Here's the drawing with two shaded views (mm, measured from the low corner). I have some questions. A direction names the side the tool comes from. Give positions to 0.01 mm unless a question says otherwise; leave off trailing zeros. Order: outer loops, then holes, each group sorted by start corner. A loop starts at its lowest first (then second) coordinate and runs counter-clockwise, first axis right, second up. Notation, with made-up numbers: M 52,25.25 L 80,25.25 A26 ccw 80,63.25 Z; hole C -32.75,-17 d11. An arc over 180 degrees is marked long. Write each question's results on one line, items separated by ' | '.
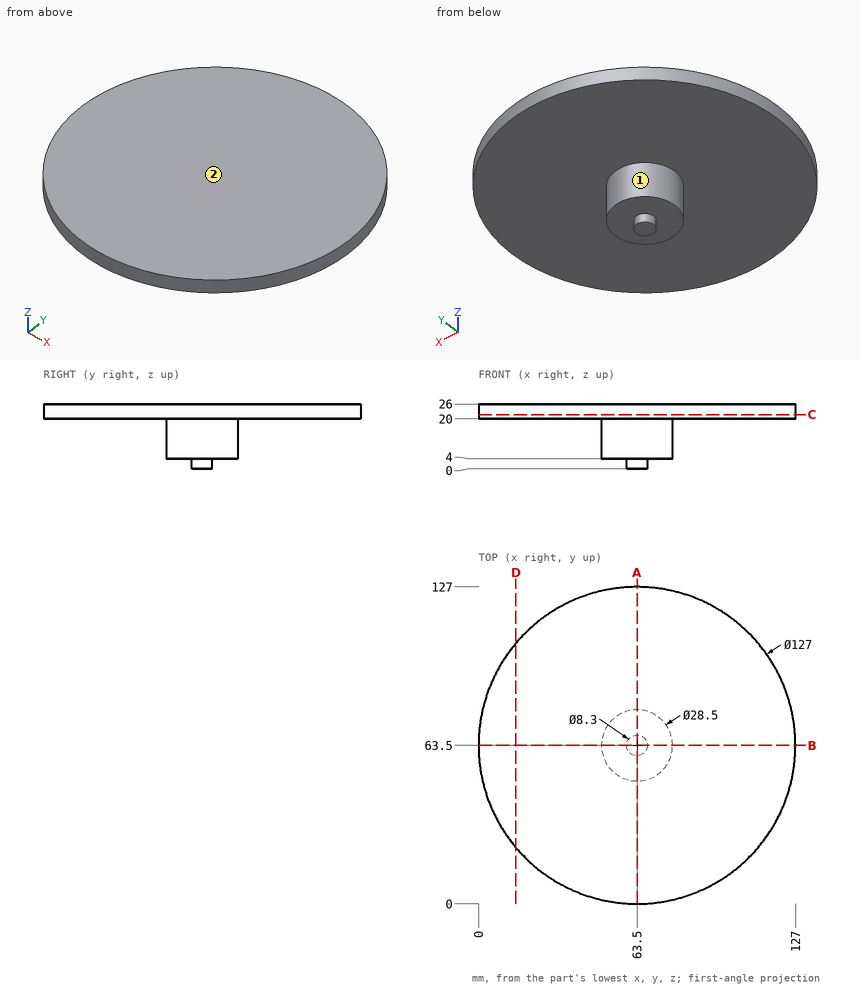
(1) I need wall thicknesses on L1, parallel to Z at x = 47, y = 80; L2, parallel to X at y = 104.5, z = 24; L3, parallel to Y at x = 59, z = 17.5. Which ranges of each line are inside material? Lowest first, please. Write a range as from..to.
Data:
L1: z = 20..26 | L2: x = 15.01..111.99 | L3: y = 49.98..77.02
(2) Imagine slicing it at A-A, the plane x = 63.5. Write out the boundary of the cut face in (y, z).
Data:
outline: M 0,20 L 49.25,20 L 49.25,4 L 59.35,4 L 59.35,0 L 67.65,0 L 67.65,4 L 77.75,4 L 77.75,20 L 127,20 L 127,26 L 0,26 Z
(3) For the marked faces 1 and 2, which set-ups out of +Z, -Z, +X, -X, +Y, -Y let a thin tool reach every point of the face, with its end or its side?
Data:
face 1: -Z | face 2: +Z, +X, -X, +Y, -Y
(4) Imagine slicing it at C-C, the plane z = 21.75. Write out the boundary of the cut face in (x, y).
Data:
outline: C 63.5,63.5 d127
(5) Will these pins go through, and if not, where does the flat tip stop? P1, Ø5, axis at x = 78.5, z = 12.5, coming from the +Y side; P2, Ø10, axis at y = 72.5, z = 3.5, coming from the -X side; P3, Ø4, axis at x = 87.5, y = 88.5, coming from the -Z side.
Data:
P1: stops at y = 70.34 | P2: stops at x = 49.83 | P3: stops at z = 20
(6) Imagine slicing it at D-D, the plane x = 15. Write out the boundary of the cut face in (y, z).
Data:
outline: M 22.51,20 L 104.49,20 L 104.49,26 L 22.51,26 Z
